Here's how the part is built. I have some questions about the finished solid (model axes, mm). Round coordinates to 2 decimals unless told otherwise and drop trailing zeros. Loops run counter-clockwise (first coordinate to the right, second up) from the corner with the lowest first, then second, coordinate; pieces in that order, holes last. Notation, with made-up numbers: (82, 50) -> (123, 50) arc R32 ccw to (123, 77) -> close; hole circle Ø2 at (-24.75, -24). An arc over 180 degrees is marked (long way). Use one line per item in the form item = value. Start each with the question number.
Item 1: I'm going to push flat-ended pins straight in: pin 1 Ø10 at (x, y) = (15, 17.5) entering from -Z; pin 2 Ø4 at (y, z) = (24, 3.5) entering from +X; pin 3 Ø21 at (x, z) = (0, 0) entering from +Y; pin 4 Ø6 at (x, z) = (4, -15.5) entering from +Y. Where does each tip first touch, or does it pass through?
Item 2: If we section it at A-A (z = -16): Write out the boundary of the cut face in (x, y).
Item 3: If we section it at B-B (z = 9): Write out the boundary of the cut face in (x, y), then the cut area to 3 significant figures.
Item 4: Thinking about a two-plate mould opening in X: for faces 1 (the face through (24.787, 19.871, -3.255)), 2 (the face through (-13.08, 23.714, 16.55)), 3 (the face through (2.85, 25.01, 20.82)), which applies, released by +X, released by -X, zero draft, split by the parting line, or undercut?
Item 5: If I drill on L1, parallel to Z at x = 0, y = 17; L2, parallel to X at y = 21, z = 12, over which ranges is the centre line in solid material (lowest first)? Write a range as [from, to].
```python
from build123d import *

# Parameters (mm, degrees)
SKETCH_1_R          = 25
EXTRUDE_1_DEPTH     = 40
SKETCH_2_R          = 17.5
CUT_EXTRUDE_1_DEPTH = 72
CUT_EXTRUDE_2_DEPTH = 38.5
SKETCH_6_R          = 21
CUT_EXTRUDE_6_DEPTH = 2
SKETCH_7_R          = 21
CUT_EXTRUDE_7_DEPTH = 2


with BuildPart() as part:
    # 草图1 → 凸台-拉伸1 (new body)
    with BuildSketch(Plane(origin=(0, 0, 0), x_dir=(1, 0, 0), z_dir=(0, 1, 0))):
        with Locations(Location((0, 0, 0), (0, 0, 270))):
            Circle(SKETCH_1_R)
    extrude(amount=EXTRUDE_1_DEPTH)

    # 草图2 → 切除-拉伸1 (cut)
    with BuildSketch(Plane(origin=(0, 40, 0), x_dir=(1, 0, 0), z_dir=(0, 1, 0))):
        with Locations(Location((0, 0, 0), (0, 0, 270))):
            Circle(SKETCH_2_R)
    extrude(amount=-CUT_EXTRUDE_1_DEPTH, mode=Mode.SUBTRACT)

    # 草图3 → 切除-拉伸2 (cut, symmetric)
    with BuildSketch(Plane.XY):
        Polygon((-25, 22), (25, 29.188898505), (25, 44.224311684), (-25, 43.752919673), align=None)
        Polygon((25, -4.224311684), (-25, -3.752919673), (-25, 18), (25, 10.811101495), align=None)
    extrude(amount=CUT_EXTRUDE_2_DEPTH, both=True, mode=Mode.SUBTRACT)

    # 草图6 → 切除-拉伸6 (cut)
    with BuildSketch(Plane(origin=(-3.605387021, 25.076074025, 0), x_dir=(0.9898214870420192, 0.14231452417067597, 0), z_dir=(-0.14231452417067594, 0.9898214870420191, 0))):
        with Locations(Location((3.642461867, 0, 0), (0, 0, 180))):
            Circle(SKETCH_6_R)
    extrude(amount=-CUT_EXTRUDE_6_DEPTH, mode=Mode.SUBTRACT)

    # 草图7 → 切除-拉伸7 (cut)
    with BuildSketch(Plane(origin=(2.029251936, 14.113789023, 0), x_dir=(0.9898214870420192, -0.14231452417067597, 0), z_dir=(-0.14231452417067594, -0.9898214870420191, 0))):
        with Locations((-2.0501191, 0)):
            Circle(SKETCH_7_R)
    extrude(amount=-CUT_EXTRUDE_7_DEPTH, mode=Mode.SUBTRACT)


solid = part.part
```
Values found:
q1.pin_1 = -22.91
q1.pin_2 = 24.95
q1.pin_3 = through
q1.pin_4 = 24.57
q2.outline = (-19.21, 17.17) -> (-13.46, 16.34) -> (-13.18, 18.32) -> (-7.09, 17.45) -> (-7.09, 22.55) -> (-13.18, 21.68) -> (-13.46, 23.66) -> (-19.21, 22.83) -> close; (7.09, 15.41) -> (13.75, 14.45) -> (13.46, 12.47) -> (19.21, 11.64) -> (19.21, 28.36) -> (13.46, 27.53) -> (13.75, 25.55) -> (7.09, 24.59) -> close
q3.outline = (-23.32, 17.76) -> (-18.78, 17.11) -> (-18.5, 19.09) -> (-15.01, 18.58) -> (-15.01, 21.42) -> (-18.5, 20.91) -> (-18.78, 22.89) -> (-23.32, 22.24) -> close; (15.01, 14.27) -> (19.07, 13.68) -> (18.78, 11.71) -> (23.32, 11.05) -> (23.32, 28.95) -> (18.78, 28.29) -> (19.07, 26.32) -> (15.01, 25.73) -> close
q3.area = 156 mm2
q4.face_1 = split by the parting line
q4.face_2 = released by -X
q4.face_3 = undercut
q5.L1 = [-25, -17.5], [17.5, 25]
q5.L2 = [-21.93, -12.74], [12.74, 21.93]
